The model under review builds one solid part; all positions refer to its coordinate system, in mm. Face numbers are marked on the shaded views. A direction names the side the tool comes from. Give positions to 0.01 mm unless a question says otherwise; leave off trailing zeros. Loops run counter-clockwise (first coordinate to the right, second up) from the corner with the lowest first, then second, coordinate; pieces in that order, holes last. Notation, with made-up numbers: M 39,-20.5 L 85,-20.5 A29 cw 85,2.5 Z; hole C 62.5,11.25 d1. An arc over 180 degrees is marked long. Return JSON: item names as keys, results as strings.
```python
from build123d import *

# Parameters (mm, degrees)
SKETCH_1_R                  = 28
SKETCH_1_R_2                = 12
EXTRUDE_1_DEPTH             = 5
HOLE_WIZARD_M4_1_AT_2_COUNT = 2
HOLE_WIZARD_M4_1_AT_2_PITCH = 39.424388736
HOLE_WIZARD_M4_1_AT_3_COUNT = 2
HOLE_WIZARD_M4_1_AT_3_PITCH = 39.424388736
HOLE_WIZARD_M4_1_AT_4_COUNT = 2
HOLE_WIZARD_M4_1_AT_4_PITCH = 18.383894388
HOLE_WIZARD_M4_1_AT_5_COUNT = 2
HOLE_WIZARD_M4_1_AT_5_PITCH = 39.424388736
HOLE_WIZARD_M4_1_AT_6_COUNT = 2
HOLE_WIZARD_M4_1_AT_6_PITCH = 18.383894388
HOLE_WIZARD_M4_1_AT_7_COUNT = 2
HOLE_WIZARD_M4_1_AT_7_PITCH = 43.5
SKETCH_4_R                  = 2
CUT_EXTRUDE_1_DEPTH         = 10


with BuildPart() as part:
    # 草图1 → 凸台-拉伸1 (new body)
    with BuildSketch(Plane.XY):
        Circle(SKETCH_1_R)
        Circle(SKETCH_1_R_2, mode=Mode.SUBTRACT)
    extrude(amount=EXTRUDE_1_DEPTH)

    # 草图3 → M4 六角凹头盖的柱孔1 (revolve, cut)
    with BuildSketch(Plane(origin=(21.75, 0, 5), x_dir=(0, -1, 0), z_dir=(1, 0, 0))):
        Polygon((0, 0), (0, 5), (2.25, 5), (2.25, 4), (4, 4), (4, 0.024142219), (4.025, 0), align=None)
    hole_wizard_m4_1 = revolve(axis=Axis((21.75, 0, 11.35), (0, 0, -1)), mode=Mode.SUBTRACT)

    # M4 六角凹头盖的柱孔1 at 2: M4 六角凹头盖的柱孔1 ×2
    with Locations(*[Vector(-0.9063077870366496, 0.42261826174070033, 0) * (i * HOLE_WIZARD_M4_1_AT_2_PITCH) for i in range(1, HOLE_WIZARD_M4_1_AT_2_COUNT)]):
        add(hole_wizard_m4_1, mode=Mode.SUBTRACT)

    # M4 六角凹头盖的柱孔1 at 3: M4 六角凹头盖的柱孔1 ×2
    with Locations(*[Vector(-0.9063077870125524, 0.42261826179237694, 0) * (i * HOLE_WIZARD_M4_1_AT_3_PITCH) for i in range(1, HOLE_WIZARD_M4_1_AT_3_COUNT)]):
        add(hole_wizard_m4_1, mode=Mode.SUBTRACT)

    # M4 六角凹头盖的柱孔1 at 4: M4 六角凹头盖的柱孔1 ×2
    with Locations(*[Vector(-0.42261826172613226, -0.9063077870434427, 0) * (i * HOLE_WIZARD_M4_1_AT_4_PITCH) for i in range(1, HOLE_WIZARD_M4_1_AT_4_COUNT)]):
        add(hole_wizard_m4_1, mode=Mode.SUBTRACT)

    # M4 六角凹头盖的柱孔1 at 5: M4 六角凹头盖的柱孔1 ×2
    with Locations(*[Vector(-0.9063077870125524, -0.42261826179237694, 0) * (i * HOLE_WIZARD_M4_1_AT_5_PITCH) for i in range(1, HOLE_WIZARD_M4_1_AT_5_COUNT)]):
        add(hole_wizard_m4_1, mode=Mode.SUBTRACT)

    # M4 六角凹头盖的柱孔1 at 6: M4 六角凹头盖的柱孔1 ×2
    with Locations(*[Vector(-0.42261826172613226, 0.9063077870434427, 0) * (i * HOLE_WIZARD_M4_1_AT_6_PITCH) for i in range(1, HOLE_WIZARD_M4_1_AT_6_COUNT)]):
        add(hole_wizard_m4_1, mode=Mode.SUBTRACT)

    # M4 六角凹头盖的柱孔1 at 7: M4 六角凹头盖的柱孔1 ×2
    with Locations(*[(-i * HOLE_WIZARD_M4_1_AT_7_PITCH, 0, 0) for i in range(1, HOLE_WIZARD_M4_1_AT_7_COUNT)]):
        add(hole_wizard_m4_1, mode=Mode.SUBTRACT)

    # 草图4 → 切除-拉伸1 (cut)
    with BuildSketch(Plane.XY):
        with Locations((0, -23)):
            Circle(SKETCH_4_R)
    extrude(amount=CUT_EXTRUDE_1_DEPTH, mode=Mode.SUBTRACT)


solid = part.part
```
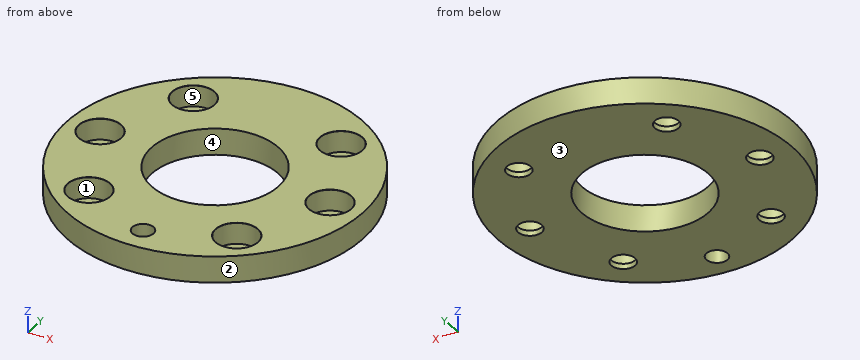
1) Consider section B-B on x = 0. Write out the cut boundary in (y, z), then the cut area to 3 significant figures.
From the geometry:
{"outline": "M -28,0 L -25,0 L -25,5 L -28,5 Z; M -21,0 L -12,0 L -12,5 L -21,5 Z; M 12,0 L 28,0 L 28,5 L 12,5 Z", "area": "140 mm²"}
2) Consider section C-C on x = 21.75. Write out the cut boundary in (y, z) (3 decimals).
From the geometry:
{"outline": "M -17.633,0 L -2.25,0 L -2.25,1 L -4,1 L -4,4.976 L -4.025,5 L -17.633,5 Z; M 2.25,0 L 17.633,0 L 17.633,5 L 4.025,5 L 4,4.976 L 4,1 L 2.25,1 Z"}
3) Tool access review of the marked faces 4 and 5: name each direction out of +Z, -Z, +X, -X, +Y, -Y from which nothing blocks a thin tool from reaching the whole face with its end or side.
From the geometry:
{"face 4": "+Z, -Z", "face 5": "+Z"}
4) Wall thickness on L1, parallel to Y at x = 0, z = 1.5; L2, parallel to Y at x = -14, z = 1.8; L3, parallel to Y at x = -11, z = 1.5: over which ranges is each line inside the solid? List them lowest first. Write a range as from..to.
From the geometry:
{"L1": "-28..-25, -21..-12, 12..28", "L2": "-24.25..-20.66, -12.66..12.66, 20.66..24.25", "L3": "-25.75..-19.33, -13.99..-4.8, 4.8..13.99, 19.33..25.75"}
5) Insertion check: pin 1 (3 mm diameter, centred on y = 14, z = 3.5, fed in from +X); pin 2 (6 mm diameter, centred on x = -13.98, y = 16.66, fed in from +Z); pin 3 (7 mm diameter, centred on x = -13.98, y = -16.66, fed in from -Z); pin 4 (3 mm diameter, centred on x = -10, z = 4.5, fed in from +Y). Each pin has a flat end and moves straight along its axis. Give the tip position at first contact, or say it passes through.
From the geometry:
{"pin 1": "x = 25.05", "pin 2": "z = 1", "pin 3": "z = 0", "pin 4": "y = 26.68"}
6) The part is to be moulded in two halves that separate along X. For the marked faces 1, 2 and 3, say which applies: released by +X, released by -X, zero draft, split by the parting line, or undercut.
From the geometry:
{"face 1": "undercut", "face 2": "split by the parting line", "face 3": "zero draft"}
7) Consider section D-D on y = 11. Write out the cut boundary in (x, z), then the cut area to 3 significant figures.
From the geometry:
{"outline": "M -25.75,0 L -4.8,0 L -4.8,5 L -25.75,5 Z; M 4.8,0 L 25.75,0 L 25.75,5 L 4.8,5 Z", "area": "210 mm²"}
8) Consider section A-A on y = 0. Write out the cut boundary in (x, z) (3 decimals).
From the geometry:
{"outline": "M -28,0 L -24,0 L -24,1 L -25.75,1 L -25.75,4.976 L -25.775,5 L -28,5 Z; M -19.5,0 L -12,0 L -12,5 L -17.725,5 L -17.75,4.976 L -17.75,1 L -19.5,1 Z; M 12,0 L 19.5,0 L 19.5,1 L 17.75,1 L 17.75,4.976 L 17.725,5 L 12,5 Z; M 24,0 L 28,0 L 28,5 L 25.775,5 L 25.75,4.976 L 25.75,1 L 24,1 Z"}
